from build123d import *

# Parameters (mm, degrees)
SKETCH_1_W          = 90
SKETCH_1_H          = 50
EXTRUDE_1_DEPTH     = 30
SKETCH_3_R          = 10.5
CUT_EXTRUDE_2_DEPTH = 108.238052948
CHAMFER_1_SIZE      = 7
SKETCH_8_R          = 18
CUT_EXTRUDE_5_DEPTH = 2
SKETCH_7_R          = 11.5
CUT_EXTRUDE_6_DEPTH = 120
SKETCH_12_W         = 15
SKETCH_12_H         = 5
CUT_EXTRUDE_8_DEPTH = 70


with BuildPart() as part:
    # 草图1 → 拉伸1 (new body)
    with BuildSketch(Plane.XY):
        with Locations((45, -25)):
            Rectangle(SKETCH_1_W, SKETCH_1_H)
    extrude(amount=EXTRUDE_1_DEPTH)

    # 草图3 → 切除-拉伸2 (cut, through all)
    with BuildSketch(Plane(origin=(0, 0, 0), x_dir=(1, 0, 0), z_dir=(0, 1, 0))):
        with Locations(Location((15, -15, 0), (0, 0, 270))):
            Circle(SKETCH_3_R)
        with Locations(Location((75, -15, 0), (0, 0, 270))):
            Circle(SKETCH_3_R)
    extrude(amount=-CUT_EXTRUDE_2_DEPTH, mode=Mode.SUBTRACT)

    # 倒角1
    chamfer_1_edges = [part.edges().sort_by_distance(p)[0] for p in [
        (90, -25, 30),
        (0, -25, 30),
        (90, -25, 0),
        (0, -25, 0),
    ]]
    chamfer(chamfer_1_edges, length=CHAMFER_1_SIZE)

    # 草图8 → 切除-拉伸5 (cut)
    with BuildSketch(Plane(origin=(0, 0, 0), x_dir=(-1, 0, 0), z_dir=(0, 0, -1))):
        with Locations((-45, -25)):
            Circle(SKETCH_8_R)
    extrude(amount=-CUT_EXTRUDE_5_DEPTH, mode=Mode.SUBTRACT)

    # 草图7 → 切除-拉伸6 (cut)
    with BuildSketch(Plane.XY.offset(30)):
        with Locations((45, -25)):
            Circle(SKETCH_7_R)
    extrude(amount=-CUT_EXTRUDE_6_DEPTH, mode=Mode.SUBTRACT)

    # 草图12 → 切除-拉伸8 (cut)
    with BuildSketch(Plane(origin=(0, 0, 0), x_dir=(-1, 0, 0), z_dir=(0, 0, -1))):
        with Locations((-45, -2.5)):
            Rectangle(SKETCH_12_W, SKETCH_12_H)
        with Locations((-45, -47.5)):
            Rectangle(SKETCH_12_W, SKETCH_12_H)
    extrude(amount=-CUT_EXTRUDE_8_DEPTH, mode=Mode.SUBTRACT)


solid = part.part
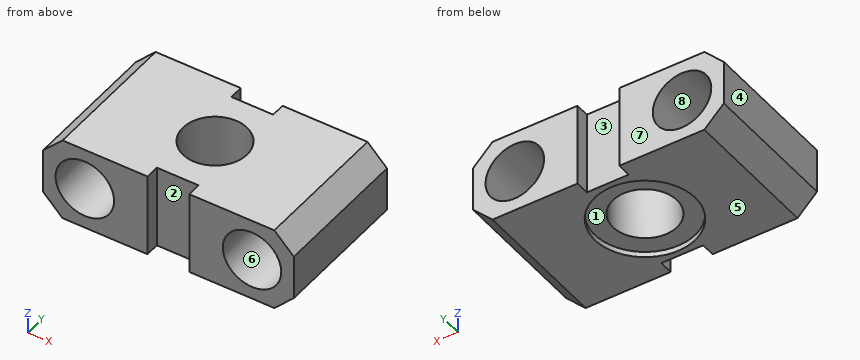
CAD build for the part. Positions are in the model's coordinates, mm. Face numbers are marked on the shaded views. A direction names the side the tool comes from. Give positions to 0.01 mm unless a question says otherwise; leave off trailing zeros. Loops run counter-clockwise (first coordinate to the right, second up) from the corner with the lowest first, then second, coordinate; pieces in that order, holes last. Notation, with made-up numbers: M 3,6 L 30,6 A24 ccw 30,24 Z; hole C 32,-11 d4. An arc over 180 degrees is marked long. One line per question, with ' | ' between items. Start each with the question number.
1. Saw through at D-D on y = -3.5. Give the cut face in (x, z), plus the area to 3 significant figures.
2. 3-axis set-ups, long thin cutter, end or side, ignore diameter. For the marked faces 1, 2, 3 and 4: which of +Z, -Z, +X, -X, +Y, -Y reach the whole face in a straight line?
3. Two-plate mould, pull along Z, no slides. Class the marked faces 5, 6, 7 and 8: pulls with the +Z half, pulls with the -Z half, needs draft (parallel to the pull), parting line crosses it, or undercut.
4. Probe L1, parallel to X at y = -40.5, z = 13; L2, parallel to X at y = -9.5, z = 23.25; L3, parallel to X at y = -15.5, z = 15. List the from-to ranges inside material, lowest first. Write a range as from..to.
5. Saw through at C-C on x = 15. Give the cut face in (y, z).
6. Saw through at A-A on y = -25. Give the cut face in (x, z), plus the area to 3 significant figures.
7. Flat gauge pins, fed straight in: pin 1 (1.5 mm diameter, centred on x = 49.5, z = 15.5, fed in from -Y); pin 2 (4.5 mm diameter, centred on x = 41.5, z = 10.5, fed in from +Y); pin 3 (18 mm diameter, centred on x = 46, y = -30, fed in from -Z). Where does each tip first touch, or does it go through?
8. Saw through at B-B on z = 14. Give the cut face in (x, y).
Result sheet:
1) outline: M 0,7 L 7,0 L 37.5,0 L 37.5,30 L 7,30 L 0,23 Z; M 52.5,0 L 83,0 L 90,7 L 90,23 L 83,30 L 52.5,30 Z; hole C 15,15 d21; hole C 75,15 d21 | area: 1,460 mm^2
2) face 1: -Z | face 2: +Z, -Z, -Y | face 3: +Z, -Z, +Y | face 4: +Z, -Z, -X, +Y, -Y
3) face 5: pulls with the -Z half | face 6: undercut | face 7: needs draft | face 8: undercut
4) L1: x = 0..4.69, 25.31..64.69, 85.31..90 | L2: x = 0.25..8.5, 21.5..68.5, 81.5..89.75 | L3: x = 0..4.5, 25.5..38.52, 51.48..64.5, 85.5..90
5) outline: M -50,0 L 0,0 L 0,4.5 L -50,4.5 Z; M -50,25.5 L 0,25.5 L 0,30 L -50,30 Z
6) outline: M 0,7 L 7,0 L 27,0 L 27,2 L 33.5,2 L 33.5,30 L 7,30 L 0,23 Z; M 56.5,2 L 63,2 L 63,0 L 83,0 L 90,7 L 90,23 L 83,30 L 56.5,30 Z; hole C 15,15 d21; hole C 75,15 d21 | area: 1,190 mm^2
7) pin 1: stops at y = -45 | pin 2: stops at y = -5 | pin 3: stops at z = 2
8) outline: M 0,-50 L 4.55,-50 L 4.55,0 L 0,0 Z; M 25.45,-50 L 37.5,-50 L 37.5,-45 L 52.5,-45 L 52.5,-50 L 64.55,-50 L 64.55,0 L 52.5,0 L 52.5,-5 L 37.5,-5 L 37.5,0 L 25.45,0 Z; M 85.45,-50 L 90,-50 L 90,0 L 85.45,0 Z; hole C 45,-25 d23
